Source: three-view drawing plus pictorial views. Frame: mm from the lowest corner of the part. A direction names the side the tool comes from. Coordinates: 2 decimals unless noted, no trailing zeros. Order: outer loops, then holes, each group sorted by start corner. A loop starts at its lowest first (then second) coordinate and runs counter-clockwise, first axis right, second up. Notation, with made-up numbers: M 85,-28 L 121,-28 A16 cw 121,-18 Z; hole C 71,-18.5 d11. An arc over 180 degrees is marked long. One line per question, with ' | ' between items.
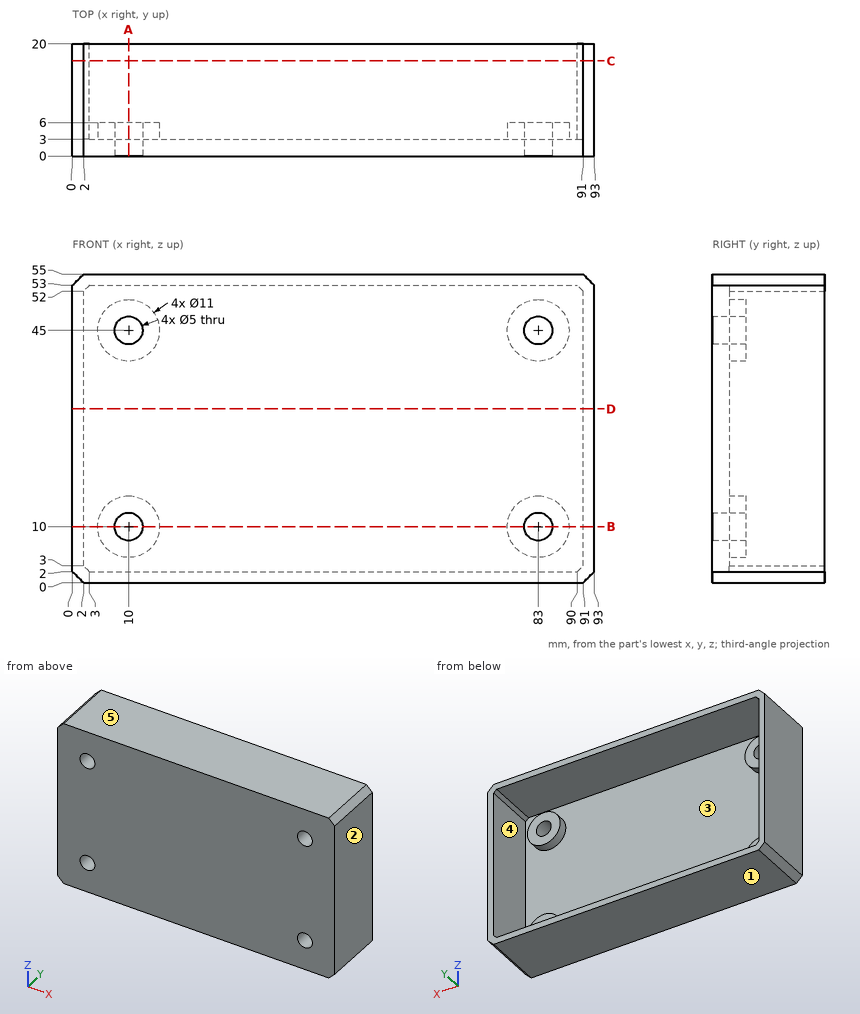
1. Draft query along Z for the marked faces 1, 2 and 3. Return one class per face: pulls with the +Z half, pulls with the -Z half, needs draft (parallel to the pull), parting line crosses it, or undercut.
Response values:
face 1: pulls with the -Z half | face 2: needs draft | face 3: undercut
2. Access query for the marked faces 4 and 5. Directions: +Z, -Z, +X, -X, +Y, -Y. A direction counts if a zero-diameter tool reaches every point of the face in a straight line with its end or side. Return the directions, or none.
Response values:
face 4: +Y | face 5: +Z, +X, -X, +Y, -Y
3. Section A-A, the plane x = 10. Output: boundary loops of the cut face in (y, z).
Response values:
outline: M 0,0 L 20,0 L 20,2 L 3,2 L 3,4.5 L 6,4.5 L 6,7.5 L 0,7.5 Z; M 0,12.5 L 6,12.5 L 6,15.5 L 3,15.5 L 3,39.5 L 6,39.5 L 6,42.5 L 0,42.5 Z; M 0,47.5 L 6,47.5 L 6,50.5 L 3,50.5 L 3,53 L 20,53 L 20,55 L 0,55 Z
4. Material intervals for line 1 (X direction, y = 1.95, z = 45); line 2 (Z direction, x = 83, y = 2.15); line 3 (Z direction, x = 21, y = 15.75), sorted ascending. Write a range as [from, to].
Response values:
line 1: x = [0, 7.5], [12.5, 80.5], [85.5, 93] | line 2: z = [0, 7.5], [12.5, 42.5], [47.5, 55] | line 3: z = [0, 2], [53, 55]
5. Section B-B, the plane z = 10. Output: boundary loops of the cut face in (x, y), and give its area (3 significant figures).
Response values:
outline: M 0,0 L 7.5,0 L 7.5,6 L 4.5,6 L 4.5,3 L 2,3 L 2,20 L 0,20 Z; M 12.5,0 L 80.5,0 L 80.5,6 L 77.5,6 L 77.5,3 L 15.5,3 L 15.5,6 L 12.5,6 Z; M 85.5,0 L 93,0 L 93,20 L 91,20 L 91,3 L 88.5,3 L 88.5,6 L 85.5,6 Z | area: 353 mm^2
6. Pin query (flat end, axial travel): P1, Ø6, axis at x = 21.5, z = 37, coming from the +Y side; P2, Ø8, axis at x = 10, z = 45, coming from the +Y side. Return the tip coordinate at first contact, or that it passes through.
Response values:
P1: stops at y = 3 | P2: stops at y = 6
7. Section C-C, the plane y = 17. Output: boundary loops of the cut face in (x, z).
Response values:
outline: M 0,2 L 2,0 L 91,0 L 93,2 L 93,53 L 91,55 L 2,55 L 0,53 Z; hole M 2,3 L 3,2 L 90,2 L 91,3 L 91,52 L 90,53 L 3,53 L 2,52 Z
8. Section D-D, the plane z = 31. Output: boundary loops of the cut face in (x, y), and give its area (3 significant figures).
Response values:
outline: M 0,0 L 93,0 L 93,20 L 91,20 L 91,3 L 2,3 L 2,20 L 0,20 Z | area: 347 mm^2
